from build123d import *

# Parameters (mm, degrees)
BOSS_EXTRUDE1_DEPTH = 20
BOSS_EXTRUDE2_DEPTH = 50
LPATTERN1_COUNT     = 2
LPATTERN1_PITCH     = 70
BOSS_EXTRUDE3_REACH = 776.125
SKETCH3_W           = 457.273423362
SKETCH3_H           = 30


with BuildPart() as part:
    # Sketch1 → Boss-Extrude1 (new body)
    with BuildSketch(Plane(origin=(0, 0, 0), x_dir=(1, 0, 0), z_dir=(0, 1, 0))):
        with BuildLine():
            Line((-228.636711681, 0), (228.636711681, 0))
            ThreePointArc((228.636711681, 0), (272.498051384, -25.996190313), (270.750281714, -76.952684821))
            Line((270.750281714, -76.952684821), (42.113570033, -434.197546823))
            ThreePointArc((42.113570033, -434.197546823), (0, -457.244862002), (-42.113570033, -434.197546823))
            Line((-42.113570033, -434.197546823), (-270.750281714, -76.952684821))
            ThreePointArc((-270.750281714, -76.952684821), (-272.498051384, -25.996190313), (-228.636711681, 0))
        make_face()
    boss_extrude1 = extrude(amount=BOSS_EXTRUDE1_DEPTH)

    # Sketch2 → Boss-Extrude2 (add)
    with BuildSketch(Plane(origin=(0, 20, 0), x_dir=(1, 0, 0), z_dir=(0, 1, 0))):
        with BuildLine():
            Line((25, -407.244862002), (25, -389.984284025))
            ThreePointArc((25, -389.984284025), (26.855525993, -403.479083858), (32.284384902, -415.972285617))
            ThreePointArc((32.284384902, -415.972285617), (72.447700685, -525.93026828), (67.470990768, -642.887877029))
            ThreePointArc((67.470990768, -642.887877029), (-29.198926208, -718.840220009), (-125.868843184, -642.887877029))
            ThreePointArc((-125.868843184, -642.887877029), (-114.073381051, -582.901412142), (-60.734106459, -553.027833807))
            ThreePointArc((-60.734106459, -553.027833807), (-55.492909619, -556.813918342), (-58.368713355, -562.604801979))
            ThreePointArc((-58.368713355, -562.604801979), (-89.779262863, -592.310875601), (-94.604026186, -635.273593035))
            ThreePointArc((-94.604026186, -635.273593035), (-29.198926208, -686.661560891), (36.20617377, -635.273593035))
            ThreePointArc((36.20617377, -635.273593035), (41.462255839, -536.500850943), (10.508220975, -442.556565834))
            ThreePointArc((10.508220975, -442.556565834), (5.87000649, -430.876676247), (4.290677946, -418.409175466))
            Line((4.290677946, -418.409175466), (4.290677946, -431.873911573))
            ThreePointArc((4.290677946, -431.873911573), (-19.134614559, -391.155532443), (25, -407.244862002))
        make_face()
    extrude(amount=BOSS_EXTRUDE2_DEPTH)

    # LPattern1: Boss-Extrude1 ×2
    with Locations(*[(0, i * LPATTERN1_PITCH, 0) for i in range(1, LPATTERN1_COUNT)]):
        add(boss_extrude1)

    # Sketch3 → Boss-Extrude3 (add, up to next)
    with BuildSketch(Plane(origin=(0, 20, 0), x_dir=(1, 0, 0), z_dir=(0, 1, 0)), mode=Mode.PRIVATE) as boss_extrude3_sk1:
        with Locations((0, -15)):
            Rectangle(SKETCH3_W, SKETCH3_H)
    boss_extrude3_tool1 = extrude(boss_extrude3_sk1.sketch, amount=BOSS_EXTRUDE3_REACH, mode=Mode.PRIVATE) - part.part
    add(boss_extrude3_tool1.solids().sort_by_distance((0, 20, 15))[0])


solid = part.part
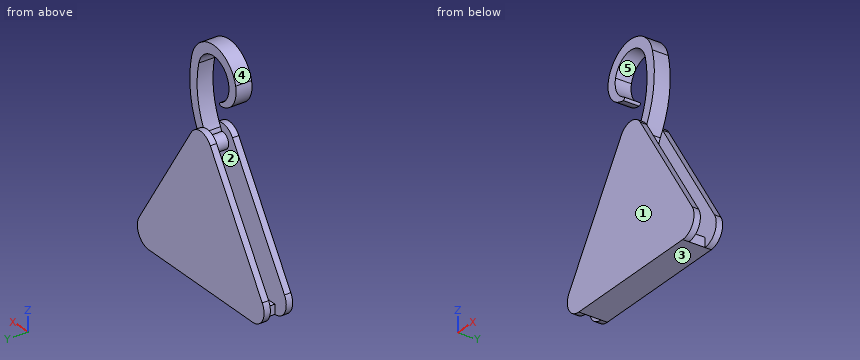
Could you check a few things on this model? Use its own coordinates, in mm. Face numbers are marked on the shaded views. A direction names the side the tool comes from. Give positions to 0.01 mm unless a question says otherwise; leave off trailing zeros. Order: outer loops, then holes, each group sorted by start corner. A loop starts at its lowest first (then second) coordinate and runs counter-clockwise, first axis right, second up.
1. Suppose I cut it at A-A (z = 311). List the corners of the cut face in (x, y) for me.
2. Will these pins go through, and if not, where does the flat tip stop? P1, Ø6, axis at x = 211, y = 22, coming from the +Z side; P2, Ø24, axis at y = 48.5, z = 14, coming from the -X side; P3, Ø8.5, axis at y = 46, z = 399.5, coming from the -X side.
3. I need wall thicknesses on L1, parallel to Y at x = 247, z = 83; L2, parallel to Z at x = -138.5, y = 35; L3, parallel to Z at x = -101.5, y = 55. Which ranges of each line are inside material? Lowest first, please.
4. Suppose I cut it at C-C (x = -144). List the corners of the cut face in (y, z) for me.
5. Suppose I cut it at D-D (z = 96.5). List the corners of the cut face in (x, y) for me.
6. We'd pull the mould along Z, two halves only. Please class the marked faces 1, 2 and 3: pulls with the +Z half, pulls with the -Z half, needs draft (parallel to the pull), parting line crosses it, or undercut.
7. For the marked faces 4 and 5, which set-ups out of +Z, -Z, +X, -X, +Y, -Y let a thin tool reach every point of the face, with its end or its side?
8. Suppose I cut it at B-B (y = 53.5). List the corners of the cut face in (x, z) for me.
Solved:
1. outline: (-120.96, 0) - (120.96, 0) - (120.96, 20) - (-120.96, 20) - close; (-120.96, 70) - (120.96, 70) - (120.96, 90) - (-120.96, 90) - close
2. P1: stops at z = 173.81
2. P2: stops at x = -228.64
2. P3: stops at x = -24.75
3. L1: y = 0 to 20, 70 to 90
3. L2: z = 0 to 30
3. L3: z = 0 to 30, 569.5 to 687.7
4. outline: (0, 0) - (90, 0) - (90, 275) - (70, 275) - (70, 30) - (20, 30) - (20, 275) - (0, 275) - close
5. outline: (-258.24, 0) - (258.24, 0) - (258.24, 20) - (-258.24, 20) - close; (-258.24, 70) - (258.24, 70) - (258.24, 90) - (-258.24, 90) - close
6. face 1: needs draft
6. face 2: undercut
6. face 3: pulls with the -Z half
7. face 4: +Z, +Y, -Y
7. face 5: +Y, -Y
8. outline: (-228.64, 0) - (228.64, 0) - (228.64, 30) - (-228.64, 30) - close; (-125.87, 642.89) arc R72.84 ccw to (-60.73, 553.03) arc R5 ccw to (-58.37, 562.6) arc R62.92 cw to (-94.6, 635.27) arc R67.32 cw to (36.21, 635.27) arc R267.82 cw to (10.51, 442.56) arc R50 ccw to (4.29, 418.41) - (4.29, 431.87) arc R25 ccw (long way) to (25, 407.24) - (25, 389.98) arc R50 cw to (32.28, 415.97) arc R300 ccw to (67.47, 642.89) arc R99.5 ccw to start
